Part model, mm, in its own coordinate system. Round coordinates to 2 decimals unless told otherwise and drop trailing zeros. Loops run counter-clockwise (first coordinate to the right, second up) from the corner with the lowest first, then second, coordinate; pieces in that order, holes last. Notation, with made-up numbers: (60, 74) -> (68, 74) arc R23 ccw to (68, 97) -> close; hole circle Ø2 at (22, 43). An arc over 180 degrees is marked (long way). Answer as a JSON object with one key per item and string values. Group by question number.
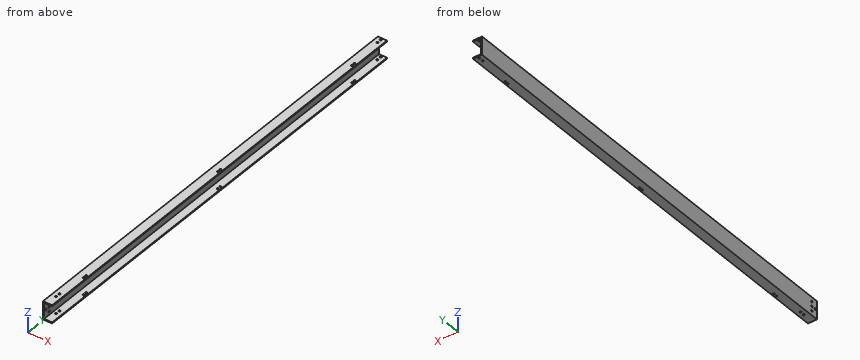
from build123d import *

# Parameters (mm, degrees)
SKETCH1_W               = 25.4
SKETCH1_H               = 50.8
SKETCH1_W_2             = 19.05
SKETCH1_H_2             = 44.45
EXTRUDE_THIN1_DEPTH     = 1244.6
SKETCH5_W               = 3.175
SKETCH5_H               = 44.45
CUT_EXTRUDE2_DEPTH      = 1245.6
SKETCH8_R               = 2.4892
CUT_EXTRUDE4_DEPTH      = 26.4
SKETCH9_R               = 2.4892
CUT_EXTRUDE5_DEPTH      = 51.8
SKETCH6_R               = 2.4892
CUT_EXTRUDE6_DEPTH      = 1
CUT_EXTRUDE6_DEPTH_BACK = 51.8
SKETCH10_R              = 2.4892
CUT_EXTRUDE7_DEPTH      = 51.8


with BuildPart() as part:
    # Sketch1 → Extrude-Thin1 (new body)
    with BuildSketch(Plane(origin=(0, 0, 0), x_dir=(1, 0, 0), z_dir=(0, 1, 0))):
        with Locations((12.7, 25.4)):
            Rectangle(SKETCH1_W, SKETCH1_H)
        with Locations((12.7, 25.4)):
            Rectangle(SKETCH1_W_2, SKETCH1_H_2, mode=Mode.SUBTRACT)
    extrude(amount=EXTRUDE_THIN1_DEPTH)

    # Sketch5 → Cut-Extrude2 (cut, through all)
    with BuildSketch(Plane(origin=(0, 1244.6, 0), x_dir=(1, 0, 0), z_dir=(0, 1, 0))):
        with Locations((23.8125, 25.4)):
            Rectangle(SKETCH5_W, SKETCH5_H)
    extrude(amount=-CUT_EXTRUDE2_DEPTH, mode=Mode.SUBTRACT)

    # Sketch8 → Cut-Extrude4 (cut, through all)
    with BuildSketch(Plane.ZY):
        with Locations((-25.4, 19.05)):
            Circle(SKETCH8_R)
        with Locations((-25.4, 6.35)):
            Circle(SKETCH8_R)
        with Locations((-38.1, 19.05)):
            Circle(SKETCH8_R)
        with Locations((-12.7, 19.05)):
            Circle(SKETCH8_R)
    extrude(amount=-CUT_EXTRUDE4_DEPTH, mode=Mode.SUBTRACT)

    # Sketch9 → Cut-Extrude5 (cut, through all)
    with BuildSketch(Plane.XY):
        with Locations((12.7, 44.45)):
            Circle(SKETCH9_R)
        with Locations((12.7, 31.75)):
            Circle(SKETCH9_R)
        with Locations((12.7, 1238.25)):
            Circle(SKETCH9_R)
        with Locations((12.7, 1225.55)):
            Circle(SKETCH9_R)
    extrude(amount=-CUT_EXTRUDE5_DEPTH, mode=Mode.SUBTRACT)

    # Sketch6 → Cut-Extrude6 (cut, two sides)
    with BuildSketch(Plane.XY) as cut_extrude6_sk:
        with Locations((19.685, 1132.205)):
            Circle(SKETCH6_R)
        with Locations((19.685, 134.62)):
            Circle(SKETCH6_R)
        with Locations((19.685, 125.095)):
            Circle(SKETCH6_R)
        with Locations((19.685, 1122.68)):
            Circle(SKETCH6_R)
    extrude(amount=CUT_EXTRUDE6_DEPTH, mode=Mode.SUBTRACT)
    extrude(cut_extrude6_sk.sketch, amount=-CUT_EXTRUDE6_DEPTH_BACK, mode=Mode.SUBTRACT)

    # Sketch10 → Cut-Extrude7 (cut, through all)
    with BuildSketch(Plane(origin=(0, 0, -50.8), x_dir=(-1, 0, 0), z_dir=(0, 0, -1))):
        with Locations((-19.685, 633.4125)):
            Circle(SKETCH10_R)
        with Locations((-19.685, 623.8875)):
            Circle(SKETCH10_R)
    extrude(amount=-CUT_EXTRUDE7_DEPTH, mode=Mode.SUBTRACT)


solid = part.part
Item 1: Drop flat-ended pins along their axis: pin 1 Ø4 at (y, z) = (6.35, -25.4) entering from -X; pin 2 Ø5 at (y, z) = (394, -27.5) entering from +X (3 decimals). Give the stop position or say it passes through.
Item 2: Drill centre lines: line 1 (X direction, y = 31, z = -48); line 2 (X direction, y = 1122.68, z = -48.5); line 3 (Y direction, x = 1.5, z = -13). Where is each one in solid material? Low to high.
Item 3: Band-saw the part on A-A, the plane y = 228. List the corners of the cut face in (x, z) (3 decimals), plus the area to 3 significant figures.
Entries:
{
 "1": {"pin 1": "through", "pin 2": "x = 3.175"},
 "2": {"line 1": "0 to 10.33, 15.07 to 25.4", "line 2": "0 to 17.2, 22.17 to 25.4", "line 3": "0 to 16.58, 21.52 to 1244.6"},
 "3": {"outline": "(0, -50.8) -> (25.4, -50.8) -> (25.4, -47.625) -> (3.175, -47.625) -> (3.175, -3.175) -> (25.4, -3.175) -> (25.4, 0) -> (0, 0) -> close", "area": "302 mm²"}
}
